Autodesk Inventor part; units mm, degrees
ref_plane "YZ Plane" through (0, 0, 0) normal (1, 0, 0) x (0, 1, 0)
ref_plane "XZ Plane" through (0, 0, 0) normal (0, 1, 0) x (-1, 0, 0)
ref_plane "XY Plane" through (0, 0, 0) normal (0, 0, 1) x (1, 0, 0)
sketch "Sketch1" plane through (0, 0, 0) normal (1, 0, 0) x (0, 1, 0)
  circle A0 centre (0, 0) radius 152.4
  line L0 (-213.36, 0) -> (213.36, 0) construction
  line L1 (0, -213.36) -> (0, 213.36) construction
  circle A1 centre (0, 139.7) radius 3.175
  circle A2 centre (0, 114.3) radius 3.175
  circle A3 centre (-69.85, 120.9837) radius 3.175
  circle A4 centre (-57.15, 98.9867) radius 3.175
  circle A5 centre (-120.9837, 69.85) radius 3.175
  circle A6 centre (-98.9867, 57.15) radius 3.175
  circle A7 centre (-139.7, 0) radius 3.175
  circle A8 centre (-114.3, 0) radius 3.175
  circle A9 centre (-120.9837, -69.85) radius 3.175
  circle A10 centre (-98.9867, -57.15) radius 3.175
  circle A11 centre (-69.85, -120.9837) radius 3.175
  circle A12 centre (-57.15, -98.9867) radius 3.175
  circle A13 centre (0, -139.7) radius 3.175
  circle A14 centre (0, -114.3) radius 3.175
  circle A15 centre (69.85, -120.9837) radius 3.175
  circle A16 centre (57.15, -98.9867) radius 3.175
  circle A17 centre (120.9837, -69.85) radius 3.175
  circle A18 centre (98.9867, -57.15) radius 3.175
  circle A19 centre (139.7, 0) radius 3.175
  circle A20 centre (114.3, 0) radius 3.175
  circle A21 centre (120.9837, 69.85) radius 3.175
  circle A22 centre (98.9867, 57.15) radius 3.175
  circle A23 centre (69.85, 120.9837) radius 3.175
  circle A24 centre (57.15, 98.9867) radius 3.175
  point P0 (0, 152.4)
  dimension "d0" = 304.8
  dimension "d1" = 12.7
  dimension "d2" = 25.4
  dimension "d3" = 6.35
  dimension "d6" = 360
extrude "Extrusion1" add sketch "Sketch1" along normal blind 1.5875
sketch "Sketch2" plane through (1.5875, 0, 0) normal (1, 0, 0) x (0, 0, -1)
  circle A0 centre (0, 0) radius 101.6
  dimension "d10" = 203.2
extrude "Extrusion2" cut sketch "Sketch2" against normal through all
properties part number "Wall" material "Aluminum 6061"
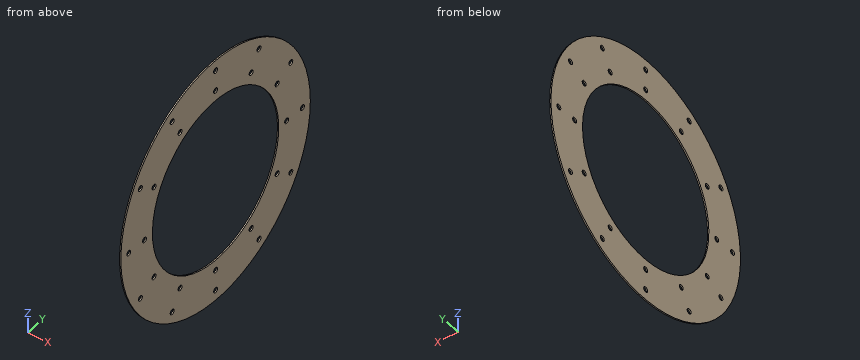
Read the model definition and answer for the solid it produces. Units are mm, in the model's axes. Coordinates: 2 decimals unless noted, no trailing zeros. Order: outer loops, then holes, each group sorted by start corner. A loop starts at its lowest first (then second) coordinate and runs counter-clockwise, first axis right, second up. Notation, with made-up numbers: M 51.25,85.5 L 103.25,85.5 A37 ccw 103.25,123.5 Z; hole C 88.5,70.25 d8. An arc over 180 degrees is marked long. Put each result on its own line as item: value. Start each with the question number.
Item 1: Section C-C, the plane z = -29 is taken. Determine the outline of the cut face in (x, y), plus the area to 3 significant figures.
Item 2: Section B-B, the plane x = 1.3 is taken. Count the separate pieces of the cut face and the enclosed holes in it, plus the area to 3 significant figures.
Item 3: Section A-A, the plane y = -34 is taken. Determine the outline of the cut face in (x, z), plus the area to 3 significant figures.
Item 4: Section D-D, the plane y = -128 is taken. Determine the outline of the cut face in (x, z), plus the area to 3 significant figures.
Item 5: Consider probe 1 along Z at (x, y) = (1.45, -68); probe 2 along Z at (x, y) = (0.7, 3.5); probe 3 along Z at (x, y) = (0.3, -120.5). Determine where each line is inside the solid, lowest interval first. Write a range as [from, to].
Item 6: Given pin 1 Ø5.5 at (y, z) = (139.7, 0) entering from -X; pin 2 Ø7.5 at (y, z) = (0, -139.7) entering from +X, each flat-ended and moving along its own axis, determine where each tip first touches the part or whether it passes through.
Computed:
1. outline: M 0,-149.62 L 1.59,-149.62 L 1.59,-97.37 L 0,-97.37 Z; M 0,97.37 L 1.59,97.37 L 1.59,149.62 L 0,149.62 Z
1. area: 166 mm2
2. separate pieces: 1
2. enclosed holes: 25
2. area: 39,800 mm2
3. outline: M 0,-148.56 L 1.59,-148.56 L 1.59,-95.74 L 0,-95.74 Z; M 0,95.74 L 1.59,95.74 L 1.59,148.56 L 0,148.56 Z
3. area: 168 mm2
4. outline: M 0,-82.71 L 1.59,-82.71 L 1.59,82.71 L 0,82.71 Z
4. area: 263 mm2
5. probe 1: z = [-136.39, -123.56], [-118.4, -75.49], [75.49, 118.4], [123.56, 136.39]
5. probe 2: z = [-152.36, -101.54], [101.54, 152.36]
5. probe 3: z = [-93.3, -72.99], [-66.71, 66.71], [72.99, 93.3]
6. pin 1: passes through
6. pin 2: stops at x = 1.59
